The model under review builds one solid part; all positions refer to its coordinate system, in mm. Coordinates: 2 decimals unless noted, no trailing zeros. Loops run counter-clockwise (first coordinate to the right, second up) from the corner with the lowest first, then second, coordinate; pieces in that order, holes last. Notation, with made-up numbers: M 49.25,-35 L 103.25,-35 A15 ccw 103.25,-16 Z; hole C 31,53 d10. An arc over 180 degrees is marked long. Write item = value, one per line. Start each with the question number.
Q1. We need section D-D on z = 9. Give the boundary of the cut face in (x, y) (1 decimal), and give its area (3 significant figures).
Q2. We need section B-B on x = 0. Give the boundary of the cut face in (y, z) (3 decimals).
Q3. Mouldability with a two-part tool opening along Y and no side actions: class faces 1 (the face through (2, 9, 0)), 2 (the face through (0, -15.875, 6)), 3 (the face through (0.553, -13.604, 6.261)) as released by +Y, released by -Y, zero draft, split by the parting line, or undercut.
Q4. Wall thickness on probe 1 along Y at (x, z) = (0, 8.5) (3 decimals); probe 2 along X at (y, z) = (11, 3.75) (3 decimals); probe 3 along Y at (x, z) = (-1, 4) (3 decimals): over which ranges is each line inside the solid? List them lowest first.
Q5. We need section A-A on z = 5.75. Give the boundary of the cut face in (x, y) (1 decimal).
Q6. We need section C-C on y = -13. Give the boundary of the cut face in (x, z) (3 decimals).
from build123d import *

# Parameters (mm, degrees)
SKETCH1_W               = 19.05
SKETCH1_H               = 31.75
BOSS_EXTRUDE1_DEPTH     = 12.7
SKETCH2_R               = 6.35
CUT_EXTRUDE1_DEPTH      = 28.86051193
F_1_4_20_TAPPED_HOLE1_D = 5.1054


with BuildPart() as part:
    # Sketch1 → Boss-Extrude1 (new body)
    with BuildSketch(Plane.XY):
        Rectangle(SKETCH1_W, SKETCH1_H)
    extrude(amount=BOSS_EXTRUDE1_DEPTH)

    # Sketch2 → Cut-Extrude1 (cut, through all)
    with BuildSketch(Plane(origin=(9.525, 0, 0), x_dir=(0, 0, -1), z_dir=(1, 0, 0))):
        Circle(SKETCH2_R)
    extrude(amount=-CUT_EXTRUDE1_DEPTH, mode=Mode.SUBTRACT)

    # 1/4-20 Tapped Hole1 (through all)
    with Locations(Plane.XY.offset(12.7)):
        with Locations((0, 11.1125), (0, -11.1125)):
            Hole(F_1_4_20_TAPPED_HOLE1_D / 2)


solid = part.part
Returned:
q1.outline = M -9.5,-15.9 L 9.5,-15.9 L 9.5,15.9 L -9.5,15.9 Z; hole C 0,-11.1 d5.1; hole C 0,11.1 d5.1
q1.area = 564 mm^2
q2.outline = M -15.875,0 L -13.665,0 L -13.665,12.7 L -15.875,12.7 Z; M -8.56,0 L -6.35,0 A6.35 cw 6.35,0 L 8.56,0 L 8.56,12.7 L -8.56,12.7 Z; M 13.665,0 L 15.875,0 L 15.875,12.7 L 13.665,12.7 Z
q3.face_1 = zero draft
q3.face_2 = released by -Y
q3.face_3 = undercut
q4.probe_1 = -15.875 to -13.665, -8.56 to 8.56, 13.665 to 15.875
q4.probe_2 = -9.525 to -2.55, 2.55 to 9.525
q4.probe_3 = -15.875 to -13.461, -8.764 to -4.932, 4.932 to 8.764, 13.461 to 15.875
q5.outline = M -9.5,-15.9 L 9.5,-15.9 L 9.5,-2.7 L -9.5,-2.7 Z; M -9.5,2.7 L 9.5,2.7 L 9.5,15.9 L -9.5,15.9 Z; hole C 0,-11.1 d5.1; hole C 0,11.1 d5.1
q6.outline = M -9.525,0 L -1.719,0 L -1.719,12.7 L -9.525,12.7 Z; M 1.719,0 L 9.525,0 L 9.525,12.7 L 1.719,12.7 Z
